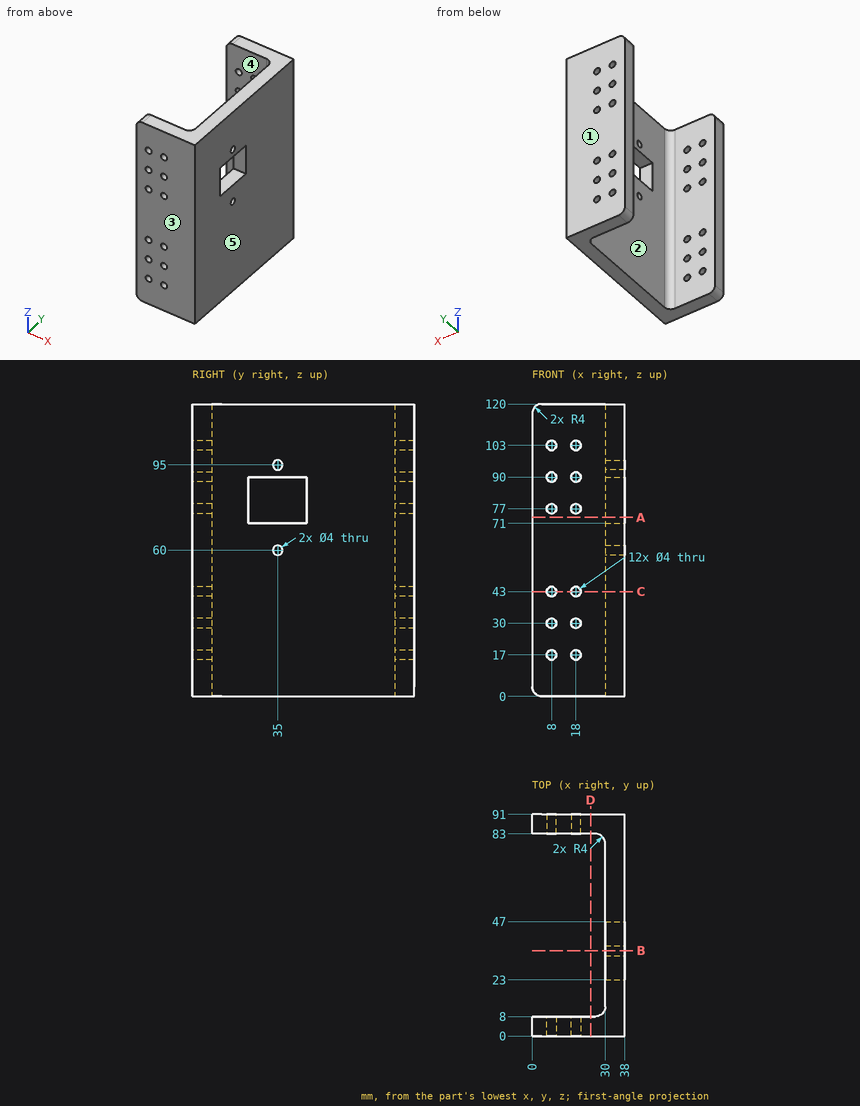
For this review, use the dimensioned drawing (mm, ordinates from the lowest corner) and the shaded views. A direction names the side the tool comes from. Round coordinates to 2 decimals unless told otherwise and drop trailing zeros. Write each loop counter-clockwise with the first axis right and the second up, starting at its lowest first coordinate (ties: lowest second). Pieces come first, ordered by that corner, then holes. Notation, with made-up numbers: M 29,55 L 57,55 A24 cw 57,81 Z; hole C -35,54.25 d1. An arc over 180 degrees is marked long. Use CSV: the item, a comma, the result in double quotes. Start each with the question number.
(1) The part is to be moulded in two halves that separate along Y. For the marked faces 3, 4 and 5, say which applies: +Y half, -Y half, draft (parallel to the pull), parting line (faces both ways), or undercut.
(2) We need section C-C, the plane z = 43. State the section outline as (x, y) points.
(3) Tool access review of the marked faces 1 and 2: name each direction out of +Z, -Z, +X, -X, +Y, -Y from which nothing blocks a thin tool from reaching the whole face with its end or side.
(4) We need section A-A, the plane z = 73.5. State the section outline as (x, y) points, then the cut area to 3 significant figures.
(5) For line 1 along Y through (x, z) = (25.5, 90); line 2 along Z through (x, y) = (32.5, 44); line 3 along X through (y, z) = (60.5, 74.5), list the stretches that pass through material, from the lowest coordinate up.
(6) Clearance check with flat-ended pins moving along their axes: P1, Ø12, axis at y = 75, z = 39, coming from the -X side; P2, Ø20, axis at y = 43, z = 84.5, coming from the -X side. State where each tip first meets the part, or that it passes through.
(7) We need section B-B, the plane y = 35. State the section outline as (x, z) points, then the cut area to 3 significant figures.
(8) We need section D-D, the plane x = 24. State the section outline as (y, z) points, then the cut area to 3 significant figures.
Findings:
1,face 3,"-Y half"
1,face 4,"undercut"
1,face 5,"draft"
2,outline,"M 0,0 L 6,0 L 6,8 L 0,8 Z; M 0,83 L 6,83 L 6,91 L 0,91 Z; M 10,0 L 16,0 L 16,8 L 10,8 Z; M 10,83 L 16,83 L 16,91 L 10,91 Z; M 20,0 L 38,0 L 38,91 L 20,91 L 20,83 L 26,83 A4 cw 30,79 L 30,12 A4 cw 26,8 L 20,8 Z"
3,face 1,"+Z, -Z, +X, -X, +Y"
3,face 2,"+Z, -Z, -X"
4,outline,"M 0,0 L 38,0 L 38,23 L 30,23 L 30,12 A4 cw 26,8 L 0,8 Z; M 0,83 L 26,83 A4 cw 30,79 L 30,47 L 38,47 L 38,91 L 0,91 Z"
4,area,"1,020 mm^2"
5,line 1,"0 to 8, 83 to 91"
5,line 2,"0 to 71, 90 to 120"
5,line 3,"30 to 38"
6,P1,"x = 29.46"
6,P2,"x = 30"
7,outline,"M 30,0 L 38,0 L 38,58 L 30,58 Z; M 30,62 L 38,62 L 38,71 L 30,71 Z; M 30,90 L 38,90 L 38,93 L 30,93 Z; M 30,97 L 38,97 L 38,120 L 30,120 Z"
7,area,"744 mm^2"
8,outline,"M 0,0 L 8,0 L 8,120 L 0,120 Z; M 83,0 L 91,0 L 91,120 L 83,120 Z"
8,area,"1,920 mm^2"
